```python
from build123d import *

# Parameters (mm, degrees)
SKETCH1_W           = 1397
SKETCH1_H           = 349.25
SKETCH1_R           = 25.4
SKETCH1_R_2         = 7.9375
BOSS_EXTRUDE1_DEPTH = 25.4


with BuildPart() as part:
    # Sketch1 → Boss-Extrude1 (new body)
    with BuildSketch(Plane.XY):
        with Locations((698.5, 174.625)):
            Rectangle(SKETCH1_W, SKETCH1_H)
        with Locations((698.5, 273.05)):
            Circle(SKETCH1_R, mode=Mode.SUBTRACT)
        with Locations((190.5, 276.225)):
            Circle(SKETCH1_R_2, mode=Mode.SUBTRACT)
        with Locations((336.55, 276.225)):
            Circle(SKETCH1_R_2, mode=Mode.SUBTRACT)
        with Locations((482.6, 276.225)):
            Circle(SKETCH1_R_2, mode=Mode.SUBTRACT)
        with Locations((631.825, 276.225)):
            Circle(SKETCH1_R_2, mode=Mode.SUBTRACT)
        with Locations(Location((1206.5, 276.225, 0), (0, 0, 180))):
            Circle(SKETCH1_R_2, mode=Mode.SUBTRACT)
        with Locations(Location((1060.45, 276.225, 0), (0, 0, 180))):
            Circle(SKETCH1_R_2, mode=Mode.SUBTRACT)
        with Locations(Location((914.4, 276.225, 0), (0, 0, 180))):
            Circle(SKETCH1_R_2, mode=Mode.SUBTRACT)
        with Locations(Location((765.175, 276.225, 0), (0, 0, 180))):
            Circle(SKETCH1_R_2, mode=Mode.SUBTRACT)
    extrude(amount=BOSS_EXTRUDE1_DEPTH)


solid = part.part
```
Geometry check sheet. Reference: the model listing, model coordinates, mm. Coordinates: 2 decimals unless noted, no trailing zeros. One line per question, with ' | ' between items. Start each with the question number.
Item 1: Material ranges on L1, parallel to Y at x = 482.6, z = 15; L2, parallel to Y at x = 336, z = 17.5; L3, parallel to X at y = 293, z = 19.5, recorded low to high. Write a range as [from, to].
Item 2: Gauge pin test, flat end, axial feed: pin 1 (18.5 mm diameter, centred on x = 482.6, y = 276.225, fed in from -Z). Record the tip position at first contact, or that the pin passes through.
Item 3: Draft check along X on faces 1 (the cylindrical face through (722.727, 280.679, 12.522)), 2 (the flat face through (689, 177, 25.4)), 3 (the flat face through (1397, 172, 13)). Enter one of: pulls with the +X half, pulls with the -X half, needs draft (parallel to the pull), parting line crosses it, or undercut.
Findings:
1) L1: y = [0, 268.29], [284.16, 349.25] | L2: y = [0, 268.31], [284.14, 349.25] | L3: x = [0, 682.78], [714.22, 1397]
2) pin 1: stops at z = 0
3) face 1: undercut | face 2: needs draft | face 3: pulls with the +X half
